Check sheet for the drawn part. Datum: minimum x, y, z corner. Units: mm. A direction names the side the tool comes from. Give positions to 0.01 mm unless a question says otherwise; leave off trailing zeros. Loops run counter-clockwise (first coordinate to the right, second up) from the corner with the lowest first, then second, coordinate; pieces in that order, holes last. Notation, with made-up numbers: (68, 35.5) - (77, 35.5) arc R25 ccw to (77, 60.5) - close; hole circle Ø1 at (5.25, -5.75). An arc over 180 degrees is marked (long way). One line per item, written item: value. Start each with the question number.
1. Scan lines: L1, parallel to Z at x = 36.83, y = 5.25; L2, parallel to X at y = 3, z = 5.08 (1 decimal); L3, parallel to X at y = 1.5, z = 6.5 (1 decimal). Record each from-to range of solid material in increasing order. Write a range as [from, to].
2. Sectioned sample at B-B (z = 5.08). Record the cut outline in (x, y).
3. Sectioned sample at C-C (x = 37). Record the cut outline in (y, z).
4. Gauge pin test, flat ends, axial feed: pin 1 (2.5 mm diameter, centred on x = 36.83, z = 33.02, fed in from +Y); pin 2 (2 mm diameter, centred on x = 52.5, y = 5.5, fed in from -Z); pin 3 (2 mm diameter, centred on x = 49, y = 1.5, fed in from +Z); pin 4 (2 mm diameter, centred on y = 5.5, z = 9, fed in from +X). Record the tip position at first contact, or that the pin passes through.
5. Sectioned sample at A-A (y = 1.5). Count the separate pieces of the cut face and the enclosed holes in it, plus the area to 3 significant figures.
6. Access from +Z, -Z, +X, -X, +Y, -Y to the whole of each face (thin tool, end or side, straight path). Record for the marked faces 1 and 2.
7. Sectioned sample at D-D (z = 33.02). Record the cut outline in (x, y), plus the area to 3 significant figures.
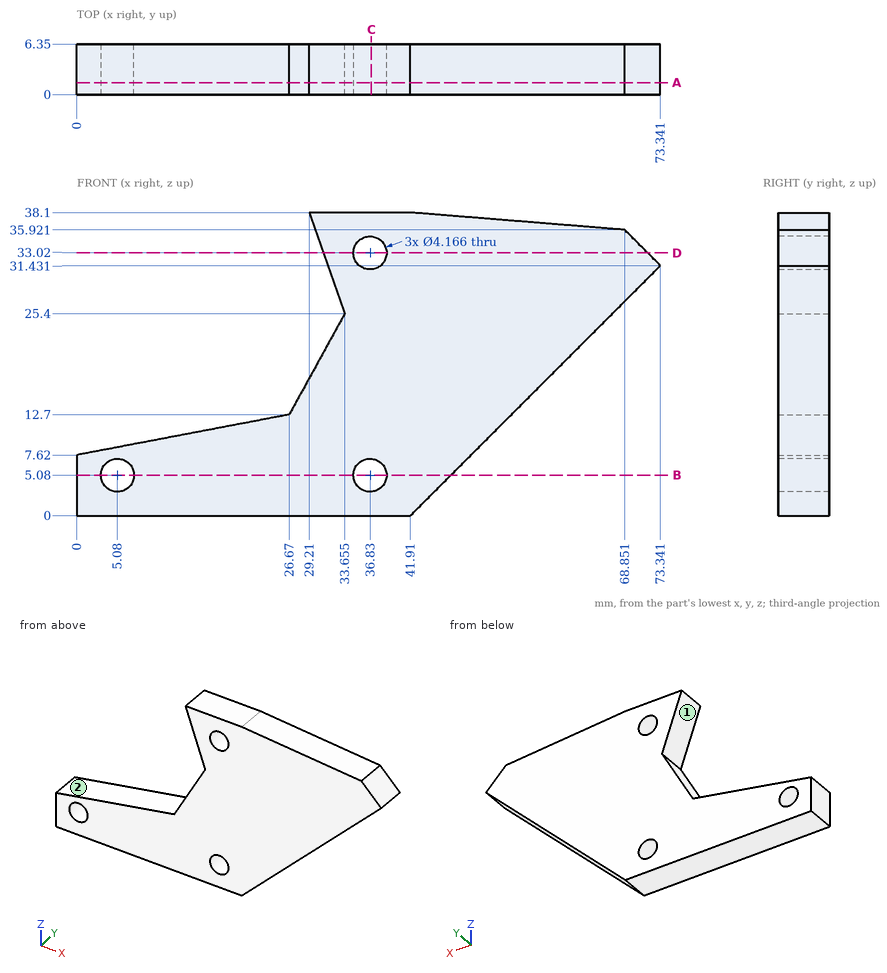
Results are:
1. L1: z = [0, 3], [7.16, 30.94], [35.1, 38.1]
1. L2: x = [0, 3], [7.2, 34.7], [38.9, 47]
1. L3: x = [0, 3.6], [6.6, 35.3], [38.4, 48.4]
2. outline: (0, 0) - (3, 0) - (3, 6.35) - (0, 6.35) - close; (7.16, 0) - (34.75, 0) - (34.75, 6.35) - (7.16, 6.35) - close; (38.91, 0) - (46.99, 0) - (46.99, 6.35) - (38.91, 6.35) - close
3. outline: (0, 0) - (6.35, 0) - (6.35, 3) - (0, 3) - close; (0, 7.16) - (6.35, 7.16) - (6.35, 30.94) - (0, 30.94) - close; (0, 35.1) - (6.35, 35.1) - (6.35, 38.1) - (0, 38.1) - close
4. pin 1: passes through
4. pin 2: stops at z = 9.59
4. pin 3: stops at z = 37.61
4. pin 4: stops at x = 51.91
5. separate pieces: 1
5. enclosed holes: 3
5. area: 1,360 mm^2
6. face 1: -X, +Y, -Y
6. face 2: +Z, -X, +Y, -Y
7. outline: (30.99, 0) - (34.75, 0) - (34.75, 6.35) - (30.99, 6.35) - close; (38.91, 0) - (71.75, 0) - (71.75, 6.35) - (38.91, 6.35) - close
7. area: 232 mm^2
